Read the model definition and answer for the solid it produces. Units are mm, in the model's axes. Coordinates: 2 decimals unless noted, no trailing zeros. Order: outer loops, then holes, each group sorted by start corner. A loop starts at its lowest first (then second) coordinate and runs counter-clockwise, first axis right, second up. Notation, with made-up numbers: M 76,-14 L 118,-14 A18 cw 118,16 Z; hole C -2,-6 d7. An arc over 180 degrees is marked long. One line per question, with ' | ' between items. Start each with the question number.
1) Find section A-A, the plane x = 0. Write down the section's boundary in (y, z).
2) Consider probe 1 along Y at (x, z) = (0, 1.95); probe 2 along Y at (x, z) = (-1, 2.4); probe 3 along X at (y, z) = (-128, 2.9). Determine where each line is inside the solid, lowest interval first.
3) Find section C-C, the plane z = 2.55. Write down the section's boundary in (x, y) (1 decimal).
4) Find section B-B, the plane y = -127. Write down the section's boundary in (x, z).
from build123d import *

# Parameters (mm, degrees)
SKETCH1_W                                = 50
SKETCH1_H                                = 300
BOSS_EXTRUDE1_DEPTH                      = 5
FILLET3_R                                = 5
CBORE_FOR_M12_HEX_HEAD_BOLT1_D           = 13.5
CBORE_FOR_M12_HEX_HEAD_BOLT1_CBORE_D     = 23.785
CBORE_FOR_M12_HEX_HEAD_BOLT1_CBORE_DEPTH = 7.5


with BuildPart() as part:
    # Sketch1 → Boss-Extrude1 (new body)
    with BuildSketch(Plane.XY):
        Rectangle(SKETCH1_W, SKETCH1_H)
    extrude(amount=BOSS_EXTRUDE1_DEPTH)

    # Fillet3
    fillet3_edges = [part.edges().sort_by_distance(p)[0] for p in [
        (-25, 150, 2.5),
        (25, 150, 2.5),
        (25, -150, 2.5),
        (-25, -150, 2.5),
    ]]
    fillet(fillet3_edges, radius=FILLET3_R)

    # CBORE for M12 Hex Head Bolt1 (through all)
    with Locations(Plane.XY.offset(5)):
        with Locations((0, 127), (0, 65), (0, -65), (0, -127)):
            CounterBoreHole(CBORE_FOR_M12_HEX_HEAD_BOLT1_D / 2, CBORE_FOR_M12_HEX_HEAD_BOLT1_CBORE_D / 2, CBORE_FOR_M12_HEX_HEAD_BOLT1_CBORE_DEPTH)


solid = part.part
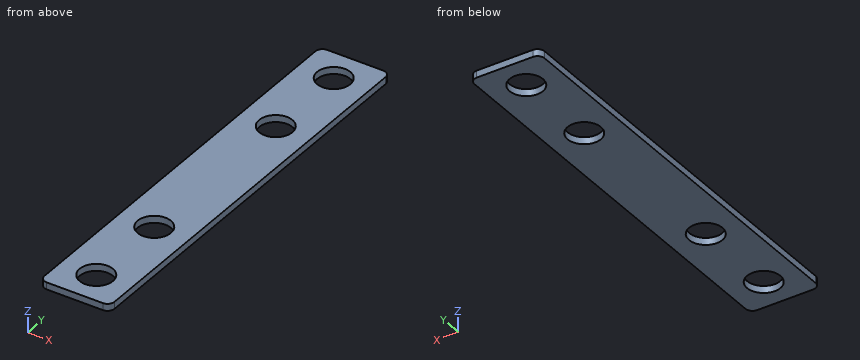
Report:
1) outline: M -150,0 L -138.89,0 L -138.89,5 L -150,5 Z; M -115.11,0 L -76.89,0 L -76.89,5 L -115.11,5 Z; M -53.11,0 L 53.11,0 L 53.11,5 L -53.11,5 Z; M 76.89,0 L 115.11,0 L 115.11,5 L 76.89,5 Z; M 138.89,0 L 150,0 L 150,5 L 138.89,5 Z
2) probe 1: y = -150 to -138.89, -115.11 to -76.89, -53.11 to 53.11, 76.89 to 115.11, 138.89 to 150 | probe 2: y = -150 to -138.85, -115.15 to -76.85, -53.15 to 53.15, 76.85 to 115.15, 138.85 to 150 | probe 3: x = -25 to -11.85, 11.85 to 25
3) outline: M -25,-145 A5 ccw -20,-150 L 20,-150 A5 ccw 25,-145 L 25,145 A5 ccw 20,150 L -20,150 A5 ccw -25,145 Z; hole C 0,-127 d23.8; hole C 0,-65 d23.8; hole C 0,65 d23.8; hole C 0,127 d23.8
4) outline: M -25,0 L -11.89,0 L -11.89,5 L -25,5 Z; M 11.89,0 L 25,0 L 25,5 L 11.89,5 Z
